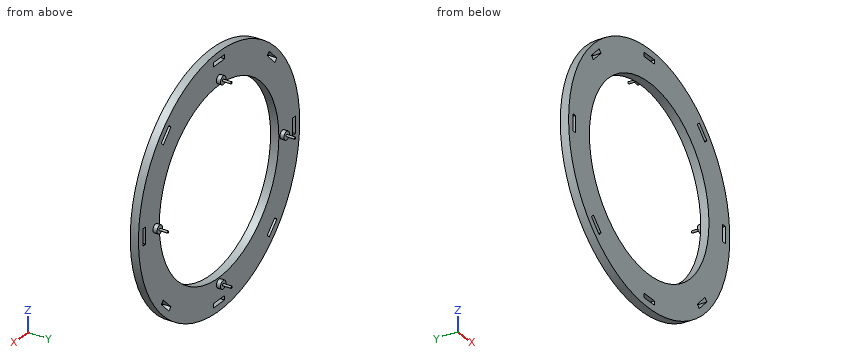
Autodesk Inventor part; units mm, degrees
ref_plane "YZ Plane" through (0, 0, 0) normal (1, 0, 0) x (0, 1, 0)
ref_plane "XZ Plane" through (0, 0, 0) normal (0, 1, 0) x (-1, 0, 0)
ref_plane "XY Plane" through (0, 0, 0) normal (0, 0, 1) x (1, 0, 0)
sketch "Sketch2" plane through (0, 0, 0) normal (0, 1, 0) x (-1, 0, 0)
  circle A0 centre (0, 0) radius 150
  dimension "d1" = 300
extrude "Extrusion1" add sketch "Sketch2" along normal blind 10
sketch "Sketch3" plane through (0, 10, 0) normal (0, 1, 0) x (1, 0, 0)
  circle A0 centre (0, 0) radius 111.25
  dimension "d4" = 222.5
sketch "Sketch4" plane through (0, 10, 0) normal (0, 1, 0) x (1, 0, 0)
  circle A0 centre (0, 0) radius 118.125
  circle A1 centre (0, 118.125) radius 1.25
  dimension "d5" = 236.25
  dimension "d6" = 2.5
extrude "Extrusion2" add sketch "Sketch4" along normal blind 15 contours A1 A0 | A0 A1 picked at (0.0501, 117.7109) picked at (0.0492, 118.5383)
sketch "Sketch5" plane through (0, 10, 0) normal (0, 1, 0) x (1, 0, 0)
  circle A0 centre (0, 118.125) radius 1.25
  circle A1 centre (0, 118.125) radius 5
  point P0 (0, 0)
  dimension "d9" = 10
extrude "Extrusion3" add sketch "Sketch5" along normal blind 5
extrude "Extrusion4" cut sketch "Sketch3" against normal blind 10
pattern_circular "Circular Pattern1" count 4 over 360 about axis through (0, -10, 0) along (0, 1, 0) of "Extrusion3", "Extrusion2"
sketch "Sketch6" plane through (0, 10, 0) normal (0, 1, 0) x (1, 0, 0)
  line L0 (0, -139.3513) -> (10, -139.3513)
  line L1 (0, -139.3513) -> (10, -139.3513) construction
  line L2 (10, -139.3513) -> (10, -141.8513)
  line L3 (10, -141.8513) -> (-10, -141.8513)
  line L4 (-10, -141.8513) -> (-10, -136.8513)
  line L5 (-10, -136.8513) -> (10, -136.8513)
  line L6 (10, -136.8513) -> (10, -141.8513)
  point P0 (0, 0)
  dimension "d17" = 10
  dimension "d18" = 0
  dimension "d19" = 2.5
  dimension "d20" = 20
  dimension "d21" = 5
extrude "Extrusion5" cut sketch "Sketch6" against normal up to surface (10 mm away)
pattern_circular "Circular Pattern2" count 8 over 360 about axis through (0, -10, 0) along (0, 1, 0) of "Extrusion5"
properties part number "TableCover"
Source: CAD feature listing. Evaluate the final solid. Frame: model axes, mm. Round coordinates to 2 decimals unless told otherwise and drop trailing zeros. Order: outer loops, then holes, each group sorted by start corner. A loop starts at its lowest first (then second) coordinate and runs counter-clockwise, first axis right, second up. Notation, with made-up numbers: (10, 48) -> (58, 48) arc R21 cw to (58, 61) -> close; hole circle Ø5 at (-20.75, 0). An arc over 180 degrees is marked (long way). Use CSV: the item, a comma, the result in double quotes.
(1) Section A-A on z = 64.5. Return the cut outline in (x, y), and give its area (3 significant figures).
Report:
outline,"(-135.42, 0) -> (-90.64, 0) -> (-90.64, 10) -> (-135.42, 10) -> close; (90.64, 0) -> (135.42, 0) -> (135.42, 10) -> (90.64, 10) -> close"
area,"896 mm^2"
(2) Ray query, L1, parallel to Z at x = 0, y = 6; L2, parallel to Z at x = 9, y = 4; L3, parallel to X at y = 8, z = -30.5. Return the intervals inside material, ascending.
Report:
L1,"-150 to -141.85, -136.85 to -111.25, 111.25 to 136.85, 141.85 to 150"
L2,"-149.73 to -141.85, -136.85 to -110.89, 110.89 to 136.85, 141.85 to 149.73"
L3,"-146.87 to -106.99, 106.99 to 146.87"
(3) First-contact query: pin 1 Ø5.5 at (x, y) = (-138.5, 6) entering from +Z; pin 2 Ø3 at (x, y) = (82.5, 4.5) entering from -Z; pin 3 Ø5 at (x, y) = (-91, 10) entering from +Z. Flat tips, straight axial feed; report the tip coordinate or a pass-through.
Report:
pin 1,"z = 63.81"
pin 2,"z = -126.25"
pin 3,"z = 121.11"
(4) Section B-B on x = 17. Return the cut outline in (y, z).
Report:
outline,"(0, -149.03) -> (10, -149.03) -> (10, -109.94) -> (0, -109.94) -> close; (0, 109.94) -> (10, 109.94) -> (10, 149.03) -> (0, 149.03) -> close"
